from build123d import *


# Not quite as in the source:
# - a feature names something its author has since deleted; it is built from what else it names


with BuildPart() as f1:
    # F0 (on Right) → F1 (revolve)
    with BuildSketch(Plane.YZ):
        Polygon((-23.5091740638, 16.747707203), (-23.5091740638, 19.747707203), (-24.0091740638, 19.747707203), (-24.5091740638, 17.747707203), (-25.0091740638, 17.747707203), (-25.0091740638, 17.247707203), (-27.0091740638, 17.247707203), (-27.0091740638, 17.747707203), (-27.5091740638, 17.747707203), (-28.0091740638, 19.747707203), (-28.5091740638, 19.747707203), (-28.5091740638, 16.747707203), (-27.0091740638, 16.747707203), (-27.0091740638, 13.122707203), (-28.5091740638, 13.122707203), (-28.5091740638, 11.247707203), (-26.0091740638, 11.247707203), (-23.5091740638, 11.247707203), (-23.5091740638, 13.122707203), (-25.0091740638, 13.122707203), (-25.0091740638, 16.747707203), align=None)
    revolve(axis=Axis((0, -33.8120413944, 9.247707203), (0, 1, 0)))


solid = f1.part
Could you check a few things on this model? Use its own coordinates, in mm. A direction names the side the tool comes from. Coordinates: 2 decimals unless noted, no trailing zeros. Order: outer loops, then holes, each group sorted by start corner. A loop starts at its lowest first (then second) coordinate and runs counter-clockwise, first axis right, second up. Notation, with made-up numbers: (31.25, 31.5) -> (81.25, 31.5) arc R34 cw to (81.25, 65.5) -> close; hole circle Ø10 at (-12.75, 74). An arc over 180 degrees is marked (long way). One line per question, with ' | ' between items.
Q1. If I drill on L1, parallel to Y at x = -4, z = 2.25; L2, parallel to Z at x = 2.5, y = -27.1; L3, parallel to Z at x = -2.5, y = -23.75, over which ranges is the centre line in solid material (lowest first)?
Return value:
L1: -28.51 to -27.01, -25.01 to -23.51 | L2: 1.12 to 2.18, 6.29 to 12.21, 16.32 to 17.37 | L3: -0.95 to 2.18, 6.29 to 12.21, 16.32 to 19.45
Q2. Imagine slicing it at A-A on y = -26. Please give me the cut outline in (x, z).
Return value:
outline: circle Ø16 at (0, 9.25); hole circle Ø4 at (0, 9.25)
Q3. On a 3-axis mill with a long thin cutter (end or side, diameter ignored), from which of +Z, -Z, +X, -X, +Y, -Y can I reach the whole of each face in a straight line? I mean faces 4 (the face through (0.09, -25.97, 7.25)), 5 (the face through (-2, -23.509, 8)), 6 (the face through (0.374, -24.763, 0.756)), 7 (the face through (-3, -27.009, 12)), 8 (the face through (0.33, -24.249, 1.755)). Say none if no direction works.
Return value:
face 4: +Y, -Y | face 5: +Z, -Z, +X, -X, +Y | face 6: none | face 7: -Y | face 8: +Y
Q4. Thinking about a two-plate mould opening in Z: for faces 1 (the face through (-3, -25.009, 6)), 2 (the face through (-6, -27.009, 15)), 3 (the face through (10.41, -23.76, 7.88)), which applies, pulls with the +Z half, pulls with the -Z half, needs draft (parallel to the pull), parting line crosses it, or undercut?
Return value:
face 1: undercut | face 2: needs draft | face 3: parting line crosses it
Q5. I'm going to push flat-ended pins straight in: P1, Ø10, axis at x = 6.5, z = 12.5, coming from the -Y side; P2, Ø2, axis at y = -24.5, z = 5, coming from the -X side. Where does each tip first touch, or does it pass through?
Return value:
P1: y = -28.51 | P2: x = -9.94
